```python
from build123d import *

# Parameters (mm, degrees)
SKETCH1_W           = 24
SKETCH1_H           = 12
BOSS_EXTRUDE1_DEPTH = 21
SKETCH2_W           = 34
SKETCH2_H           = 12
SKETCH2_R           = 1
BOSS_EXTRUDE2_DEPTH = 1.5
SKETCH3_W           = 15
SKETCH3_H           = 12
BOSS_EXTRUDE3_DEPTH = 5
SKETCH4_R           = 2
BOSS_EXTRUDE4_DEPTH = 4


with BuildPart() as part:
    # Sketch1 → Boss-Extrude1 (new body)
    with BuildSketch(Plane.XY):
        with Locations((12, -6)):
            Rectangle(SKETCH1_W, SKETCH1_H)
    extrude(amount=BOSS_EXTRUDE1_DEPTH)

    # Sketch2 → Boss-Extrude2 (add)
    with BuildSketch(Plane.XY.offset(6)):
        with Locations((12, -6)):
            Rectangle(SKETCH2_W, SKETCH2_H)
        with Locations((-2.5, -2)):
            Circle(SKETCH2_R, mode=Mode.SUBTRACT)
        with Locations((26.5, -2)):
            Circle(SKETCH2_R, mode=Mode.SUBTRACT)
        with Locations((26.5, -6)):
            Circle(SKETCH2_R, mode=Mode.SUBTRACT)
        with Locations((26.5, -10)):
            Circle(SKETCH2_R, mode=Mode.SUBTRACT)
        with Locations((-2.5, -6)):
            Circle(SKETCH2_R, mode=Mode.SUBTRACT)
        with Locations((-2.5, -10)):
            Circle(SKETCH2_R, mode=Mode.SUBTRACT)
    extrude(amount=-BOSS_EXTRUDE2_DEPTH)

    # Sketch3 → Boss-Extrude3 (add)
    with BuildSketch(Plane(origin=(0, 0, 0), x_dir=(-1, 0, 0), z_dir=(0, 0, -1))):
        with Locations((-16.5, -6)):
            Rectangle(SKETCH3_W, SKETCH3_H)
    extrude(amount=BOSS_EXTRUDE3_DEPTH)

    # Sketch4 → Boss-Extrude4 (add)
    with BuildSketch(Plane(origin=(0, 0, -5), x_dir=(-1, 0, 0), z_dir=(0, 0, -1))):
        with Locations((-17, -6)):
            Circle(SKETCH4_R)
    extrude(amount=BOSS_EXTRUDE4_DEPTH)


solid = part.part
```
Can you work these out from the model? Positions are in its coordinate system, mm. A direction names the side the tool comes from. Coordinates: 2 decimals unless noted, no trailing zeros. Order: outer loops, then holes, each group sorted by start corner. A loop starts at its lowest first (then second) coordinate and runs counter-clockwise, first axis right, second up. Notation, with made-up numbers: (76.25, -17) -> (81.25, -17) arc R28 ccw to (81.25, 16) -> close; hole circle Ø1 at (-2.75, -7.5). An arc over 180 degrees is marked (long way). Write each question's results on one line, items separated by ' | '.
Item 1: I want a section at D-D, the plane x = 17. Write out the boundary of the cut face in (y, z).
Results are:
outline: (-12, -5) -> (-8, -5) -> (-8, -9) -> (-4, -9) -> (-4, -5) -> (0, -5) -> (0, 21) -> (-12, 21) -> close
Item 2: I want a section at A-A, the plane y = -6. Write out the boundary of the cut face in (x, z).
Results are:
outline: (-5, 4.5) -> (-3.5, 4.5) -> (-3.5, 6) -> (-5, 6) -> close; (-1.5, 4.5) -> (0, 4.5) -> (0, 0) -> (9, 0) -> (9, -5) -> (15, -5) -> (15, -9) -> (19, -9) -> (19, -5) -> (24, -5) -> (24, 4.5) -> (25.5, 4.5) -> (25.5, 6) -> (24, 6) -> (24, 21) -> (0, 21) -> (0, 6) -> (-1.5, 6) -> close; (27.5, 4.5) -> (29, 4.5) -> (29, 6) -> (27.5, 6) -> close
Item 3: I want a section at C-C, the plane y = -8.5. Write out the boundary of the cut face in (x, z).
Results are:
outline: (-5, 4.5) -> (0, 4.5) -> (0, 0) -> (9, 0) -> (9, -5) -> (24, -5) -> (24, 4.5) -> (29, 4.5) -> (29, 6) -> (24, 6) -> (24, 21) -> (0, 21) -> (0, 6) -> (-5, 6) -> close
Item 4: If we mould it in two halves opening along X, with no side actions, what happens to faces 6 (the face through (26.37, -9.01, 5.26)), 7 (the face through (24, -6, 0)), 8 (the face through (-1, -6, 6))? For each: +X half, -X half, draft (parallel to the pull), parting line (faces both ways), or undercut.
Results are:
face 6: undercut | face 7: +X half | face 8: draft
Item 5: I'm going to push flat-ended pins straight in: pin 1 Ø5.5 at (y, z) = (-4.5, -2) entering from -X; pin 2 Ø1.8 at (x, y) = (26.5, -10) entering from -Z; pin 3 Ø2 at (x, y) = (17.5, -9.5) entering from -Z; pin 4 Ø3 at (x, y) = (-1, -1.5) entering from +Z. Where does each tip first touch, or does it pass through?
Results are:
pin 1: x = 0 | pin 2: through | pin 3: z = -5 | pin 4: z = 21
Item 6: If I drill on line 1 along Y through (x, z) = (-2.5, 5.4); line 2 along X through (y, z) = (-6.5, 8); line 3 along Z through (x, y) = (23, -4), over which ranges is the centre line in solid material (lowest first)?
Results are:
line 1: -12 to -11, -9 to -7, -5 to -3, -1 to 0 | line 2: 0 to 24 | line 3: -5 to 21
Item 7: Which directions (+Z, -Z, +X, -X, +Y, -Y) give clear straight access to the entire face, cutting with the end or side of a thin tool? Please do faces 1 (the face through (18.6, -7.2, -7)), 2 (the face through (28, -6, 4.5)), 3 (the face through (0, -6, 2)), 4 (the face through (-3.3, -2.6, 5.3)), 5 (the face through (28, -6, 6)).
Results are:
face 1: -Z | face 2: -Z, +X, +Y, -Y | face 3: -Z, -X, +Y, -Y | face 4: +Z, -Z | face 5: +Z, +X, +Y, -Y
Item 8: I want a section at B-B, the plane x = 26.5. Write out the boundary of the cut face in (y, z), then the cut area to 3 significant figures.
Results are:
outline: (-12, 4.5) -> (-11, 4.5) -> (-11, 6) -> (-12, 6) -> close; (-9, 4.5) -> (-7, 4.5) -> (-7, 6) -> (-9, 6) -> close; (-5, 4.5) -> (-3, 4.5) -> (-3, 6) -> (-5, 6) -> close; (-1, 4.5) -> (0, 4.5) -> (0, 6) -> (-1, 6) -> close | area: 9.00 mm²
